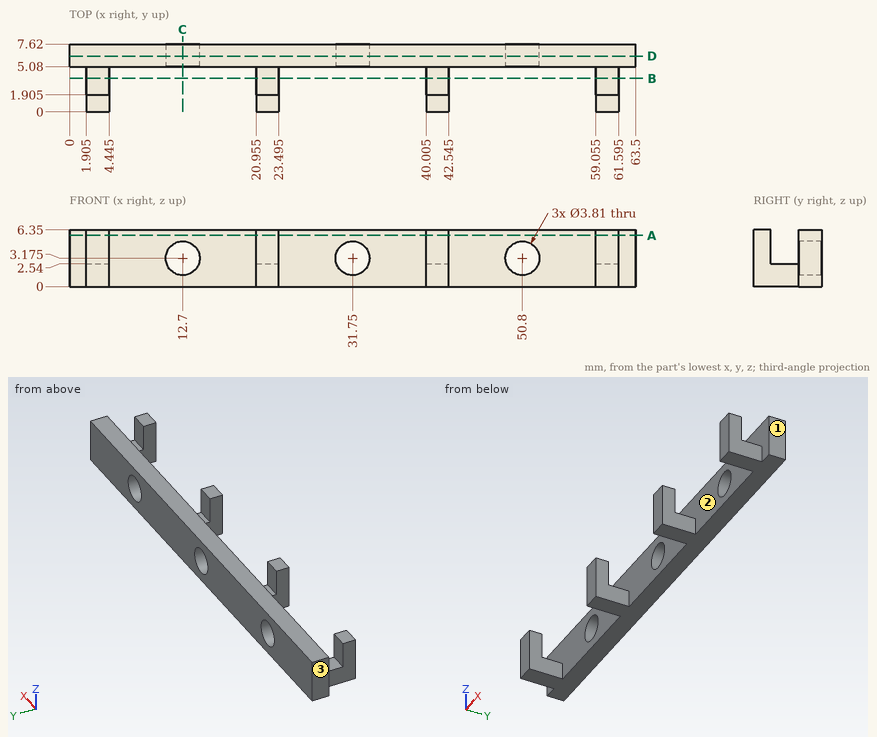
Design review of the part shown in the three views and the two pictorial views. Dimensions are in mm from the part's minimum x, y and z. Round coordinates to 2 decimals unless told otherwise and drop trailing zeros. Write each loop counter-clockwise with the first axis right and the second up, starting at its lowest first coordinate (ties: lowest second). Pieces come first, ordered by that corner, then holes.
Item 1: We need section C-C on x = 12.7. Write out the cut boundary in (y, z).
Item 2: The part is to be moulded in two halves that separate along X. For the marked faces 1, 2 and 3, say which applies: +X half, -X half, draft (parallel to the pull), parting line (faces both ways), or undercut.
Item 3: For probe 1 along X at (y, z) = (3.5, 1.25) (3 decimals); probe 2 along Z at (x, y) = (12.7, 6); probe 3 along Y at (x, z) = (47, 0.5), list the stretches that pass through material, from the lowest coordinate up.
Item 4: We need section B-B on y = 3.75. Write out the cut boundary in (x, z) (3 decimals).
Item 5: Clearance check with flat-ended pins moving along their axes: pin 1 Ø2 at (x, y) = (61, 3.5) entering from +Z; pin 2 Ø1 at (x, z) = (46, 4) entering from -Y. State where each tip first meets the part, or that it passes through.
Item 6: We need section A-A on z = 5.75. Write out the cut boundary in (x, y) (3 decimals), and give its area (3 significant figures).
Item 7: We need section D-D on y = 6.25. Write out the cut boundary in (x, z) (3 decimals), and give its area (3 significant figures).
Returned:
1. outline: (5.08, 0) - (7.62, 0) - (7.62, 1.27) - (5.08, 1.27) - close; (5.08, 5.08) - (7.62, 5.08) - (7.62, 6.35) - (5.08, 6.35) - close
2. face 1: +X half
2. face 2: undercut
2. face 3: -X half
3. probe 1: x = 1.905 to 4.445, 20.955 to 23.495, 40.005 to 42.545, 59.055 to 61.595
3. probe 2: z = 0 to 1.27, 5.08 to 6.35
3. probe 3: y = 5.08 to 7.62
4. outline: (1.905, 0) - (4.445, 0) - (4.445, 2.54) - (1.905, 2.54) - close; (20.955, 0) - (23.495, 0) - (23.495, 2.54) - (20.955, 2.54) - close; (40.005, 0) - (42.545, 0) - (42.545, 2.54) - (40.005, 2.54) - close; (59.055, 0) - (61.595, 0) - (61.595, 2.54) - (59.055, 2.54) - close
5. pin 1: stops at z = 2.54
5. pin 2: stops at y = 5.08
6. outline: (0, 5.08) - (63.5, 5.08) - (63.5, 7.62) - (0, 7.62) - close; (1.905, 0) - (4.445, 0) - (4.445, 1.905) - (1.905, 1.905) - close; (20.955, 0) - (23.495, 0) - (23.495, 1.905) - (20.955, 1.905) - close; (40.005, 0) - (42.545, 0) - (42.545, 1.905) - (40.005, 1.905) - close; (59.055, 0) - (61.595, 0) - (61.595, 1.905) - (59.055, 1.905) - close
6. area: 181 mm2
7. outline: (0, 0) - (63.5, 0) - (63.5, 6.35) - (0, 6.35) - close; hole circle Ø3.81 at (12.7, 3.175); hole circle Ø3.81 at (31.75, 3.175); hole circle Ø3.81 at (50.8, 3.175)
7. area: 369 mm2
